The model under review builds one solid part; all positions refer to its coordinate system, in mm. A direction names the side the tool comes from. Give positions to 0.01 mm unless a question says otherwise; leave off trailing zeros. Order: outer loops, then holes, each group sorted by start corner. A loop starts at its lowest first (then second) coordinate and runs counter-clockwise, first axis right, second up. Notation, with made-up numbers: (-25, 11) - (10, 11) arc R28 cw to (10, 43) - close; hole circle Ø7 at (11, 67.5). An arc over 180 degrees is marked (long way). Use CSV: the item, a comma, the result in double quotes. Start each with the question number.
1. Machinability: for faces 1 (the flat face through (-0.635, 8, 0)), 2 (the flat face through (22.86, 18.7, -1.4)), 3 (the flat face through (-0.009, 8.219, -1.134)), 4 (the flat face through (44, 16.243, 3)), which of the approach directions +Z, -Z, +X, -X, +Y, -Y give a long, thin tool a straight path to every point of the face, cutting with its end or side? Answer none if there is none.
2. To check wall thickness, follow line 1 (X direction, y = 8.75, z = -0.25) (3 decimals); line 2 (X direction, y = 14, z = 2); line 3 (Z direction, x = 23, y = 8) (3 decimals). State the ranges of each line that lie inside material, in increasing order. Write a range as [from, to].
3. Take a section at A-A, the plane x = 41. State the section outline as (y, z) points (3 decimals), then the cut area to 3 significant figures.
4. Take a section at B-B, the plane y = 9.5. State the section outline as (x, z) points (3 decimals), then the cut area to 3 significant figures.
5. Take a section at C-C, the plane y = 13. State the section outline as (x, z) points (3 decimals).
6. For pin 1 (1.5 mm diameter, centred on x = 7, y = 19, fed in from +Z) (3 decimals); pin 2 (1.5 mm diameter, centred on x = 10.5, y = 16, fed in from -Z) (3 decimals); pin 3 (2 mm diameter, centred on y = 12, z = 3, fed in from -X); pin 4 (1.3 mm diameter, centred on y = 11.5, z = 2.5, fed in from +X), all flat-tipped, find the tip position at first contact; note any pin that passes through.
7. Take a section at D-D, the plane x = 15. State the section outline as (y, z) points (3 decimals).
8. Draft analysis for pull direction X (two halves, no side actions). For faces 5 (the flat face through (51, 5.715, -1.3)), 6 (the cylindrical face through (52.385, 8.084, 3.54)), 7 (the cylindrical face through (25.053, 20.635, 3.54)), state which applies: released by +X, released by -X, zero draft, split by the parting line, or undercut.
Autodesk Inventor part; units mm, degrees
ref_plane "YZ Plane" through (0, 0, 0) normal (1, 0, 0) x (0, 1, 0)
ref_plane "XZ Plane" through (0, 0, 0) normal (0, 1, 0) x (-1, 0, 0)
ref_plane "XY Plane" through (0, 0, 0) normal (0, 0, 1) x (1, 0, 0)
sketch "Sketch1" plane through (0, 0, 0) normal (0, 0, 1) x (1, 0, 0)
  line L0 (0, 0) -> (50.8, 0)
  line L1 (50.8, 0) -> (50.8, 19.05)
  line L2 (50.8, 19.05) -> (0, 19.05)
  line L3 (0, 19.05) -> (0, 0)
  line L4 (0, 0) -> (0, -2.54)
  line L5 (0, -2.54) -> (-2.54, -2.54)
  line L6 (-2.54, -2.54) -> (-2.54, 19.05)
  line L7 (-2.54, 19.05) -> (-2.54, 21.59)
  line L8 (-2.54, 21.59) -> (53.34, 21.59)
  line L9 (53.34, 21.59) -> (53.34, -2.54)
  line L10 (53.34, -2.54) -> (0, -2.54)
  dimension "d0" = 50.8
  dimension "d1" = 19.05
  dimension "d2" = 50.8
  dimension "d3" = 2.54
  dimension "d4" = 2.54
  dimension "d5" = 2.54
  dimension "d6" = 55.88
extrude "Extrusion1" add sketch "Sketch1" along normal blind 1.905
sketch "Sketch2" plane through (0, 0, 1.905) normal (0, 0, 1) x (1, 0, 0)
  line L0 (-2.54, -2.54) -> (-2.54, 21.59)
  line L1 (-2.54, 21.59) -> (53.34, 21.59)
  line L2 (53.34, 21.59) -> (-2.54, 21.59)
  line L3 (53.34, 21.59) -> (53.34, -2.54)
  line L4 (53.34, -2.54) -> (-2.54, -2.54)
  line L5 (-2.54, -2.54) -> (53.34, -2.54)
  point P0 (0, 0)
extrude "Extrusion2" add sketch "Sketch2" along normal blind 2.54
sketch "Sketch3" plane through (0, 0, 0) normal (0, 0, -1) x (-1, 0, 0)
  line L0 (0, 0) -> (2.54, 0)
  line L1 (2.54, 21.59) -> (2.54, -2.54)
  line L2 (2.54, 0) -> (2.54, 19.05)
  line L3 (2.54, 0) -> (0.635, 0)
  line L4 (0.635, 0) -> (0.635, 19.05)
  line L5 (0.635, 19.05) -> (0, 19.05)
  line L6 (0, 19.05) -> (0, 0)
  line L7 (0, 0) -> (-50.8, 0)
  line L8 (0, 19.05) -> (0.635, 19.05)
  line L9 (-50.8, 0) -> (-51.435, 0)
  line L10 (-51.435, 0) -> (-51.435, 19.05)
  line L11 (-51.435, 19.05) -> (-50.8, 19.05)
  line L12 (-50.8, 19.05) -> (-50.8, 0)
  dimension "d11" = 1.905
  dimension "d12" = 0.635
  dimension "d13" = 19.05
extrude "Extrusion3" cut sketch "Sketch3" against normal blind 1.905
sketch "Sketch4" plane through (0, 0, 0) normal (0, 0, -1) x (-1, 0, 0)
  line L0 (2.54, -2.54) -> (-53.34, -2.54)
  line L1 (0, 0) -> (-51.435, 0)
  line L2 (-51.435, 0) -> (-51.435, 19.05)
  line L3 (-51.435, 0) -> (-51.435, -2.54)
  line L4 (-51.435, -2.54) -> (0, -2.54)
  line L5 (0.635, 0) -> (0.635, -2.54)
  line L6 (0.635, 0) -> (0, 0)
  line L7 (0.635, 0) -> (-51.435, 0)
  line L8 (0.635, -2.54) -> (0, -2.54)
extrude "Extrusion4" cut sketch "Sketch4" against normal blind 1.905
sketch "Sketch5" plane through (0, 0, 4.445) normal (0, 0, 1) x (1, 0, 0)
  line L0 (-2.54, 21.59) -> (7.62, 21.59)
  line L1 (53.34, 21.59) -> (-2.54, 21.59)
  line L2 (7.62, 21.59) -> (7.62, 11.43)
  line L3 (-2.54, 21.59) -> (5.08, 21.59)
  line L4 (5.08, 21.59) -> (5.08, 13.97)
  line L5 (5.08, 13.97) -> (7.62, 13.97)
  line L6 (5.08, 13.97) -> (5.08, 11.43)
  line L7 (5.08, 11.43) -> (7.62, 11.43)
  line L8 (-2.54, 21.59) -> (26.67, 21.59)
  line L9 (-2.54, 21.59) -> (19.05, 21.59)
  line L10 (19.05, 10.795) -> (26.67, 10.795)
  line L11 (26.67, 18.415) -> (19.05, 18.415)
  line L12 (26.67, 21.59) -> (29.21, 21.59)
  line L13 (19.05, 21.59) -> (21.59, 21.59)
  line L14 (21.59, 10.795) -> (29.21, 10.795)
  line L15 (29.21, 10.795) -> (29.21, 21.59)
  line L16 (26.67, 18.415) -> (29.21, 18.415)
  line L17 (21.59, 21.59) -> (21.59, 18.415)
  line L18 (29.21, 18.415) -> (21.59, 18.415)
  line L19 (21.59, 18.415) -> (21.59, 10.795)
  line L20 (53.34, 21.59) -> (40.64, 21.59)
  line L21 (40.64, 21.59) -> (40.64, 8.89)
  line L22 (53.34, 21.59) -> (47.625, 21.59)
  line L23 (47.625, 21.59) -> (47.625, 15.875)
  line L24 (47.625, 15.875) -> (40.64, 15.875)
  line L25 (47.625, 15.875) -> (47.625, 8.89)
  line L26 (47.625, 8.89) -> (40.64, 8.89)
  point P0 (0, 0)
  dimension "d18" = 10.16
  dimension "d19" = 10.16
  dimension "d20" = 7.62
  dimension "d21" = 7.62
  dimension "d22" = 29.21
  dimension "d23" = 21.59
  dimension "d24" = 10.795
  dimension "d25" = 3.175
  dimension "d26" = 2.54
  dimension "d27" = 2.54
  dimension "d28" = 12.7
  dimension "d29" = 12.7
  dimension "d30" = 5.715
extrude "Extrusion5" cut sketch "Sketch5" against normal blind 2.54 contours L5 L2 L7 L6 | L25 L26 L21 L24 | L15 L14 L10 L19 L11 L16
move faces "Move1" translate (0, -2.54, 0) faces at (26.67, 18.415, 3.5983)
move faces "Move2" translate (0, 0, -0.635) faces at (34.0783, 20.7433, 0)
sketch "Sketch6" plane through (53.34, 21.59, -0.635) normal (0, 0, -1) x (-1, 0, 0)
  line L0 (1.905, -2.54) -> (1.905, -13.335)
  line L1 (1.905, -24.13) -> (1.905, -2.54)
  line L2 (1.905, -13.335) -> (1.905, -10.795)
  line L3 (1.905, -13.335) -> (1.905, -15.875)
  line L4 (1.905, -15.875) -> (3.175, -15.875)
  line L5 (3.175, -15.875) -> (3.175, -10.795)
  line L6 (3.175, -10.795) -> (1.905, -10.795)
  line L7 (1.905, -2.54) -> (27.94, -2.54)
  line L8 (1.905, -2.54) -> (53.975, -2.54)
  line L9 (27.94, -2.54) -> (30.48, -2.54)
  line L10 (27.94, -2.54) -> (25.4, -2.54)
  line L11 (25.4, -2.54) -> (25.4, -3.81)
  line L12 (25.4, -3.81) -> (30.48, -3.81)
  line L13 (30.48, -3.81) -> (30.48, -2.54)
  line L14 (53.975, -2.54) -> (53.975, -13.335)
  line L15 (53.975, -2.54) -> (53.975, -24.13)
  line L16 (53.975, -13.335) -> (53.975, -10.795)
  line L17 (53.975, -10.795) -> (52.705, -10.795)
  line L18 (52.705, -10.795) -> (52.705, -15.875)
  line L19 (52.705, -15.875) -> (53.975, -15.875)
  line L20 (53.975, -15.875) -> (53.975, -10.795)
  point P0 (53.34, -21.59)
  dimension "d39" = 10.795
  dimension "d40" = 2.54
  dimension "d41" = 2.54
  dimension "d42" = 5.08
  dimension "d43" = 26.035
  dimension "d44" = 2.54
  dimension "d45" = 2.54
  dimension "d46" = 1.27
  dimension "d47" = 5.08
  dimension "d48" = 10.795
  dimension "d49" = 2.54
  dimension "d51" = 1.27
  dimension "d52" = 5.08
extrude "Extrusion6" add sketch "Sketch6" against normal blind 0.889
move faces "Move3" translate (0, 0, -0.381) faces at (26.2467, 20.7433, -0.635)
move faces "Move4" translate (0, 0, -0.762) faces at (24.5533, 20.7433, -1.016)
sketch "Sketch10" plane through (50.165, 10.795, 0.254) normal (0, 1, 0) x (1, 0, 0)
  line L0 (1.27, 2.032) -> (1.27, 0)
  line L1 (1.27, 2.032) -> (1.27, 0.762)
  line L2 (0, 2.032) -> (0, 0)
  line L3 (1.27, 0.762) -> (0, 2.032)
  line L4 (1.27, 0) -> (0, 0)
  line L5 (0, 2.032) -> (0, 0)
  line L6 (0, 0) -> (1.27, 0)
  line L7 (1.27, 0) -> (1.27, 0.762)
  point P0 (-50.165, 0.254)
  dimension "d70" = 1.27
extrude "Extrusion10" cut sketch "Sketch10" against normal blind 25.4
sketch "Sketch11" plane through (22.86, 17.78, 0.254) normal (-1, 0, 0) x (0, 0, 1)
  line L0 (-2.032, 1.27) -> (-0.762, 1.27)
  line L1 (-2.032, 1.27) -> (0, 1.27)
  line L2 (-2.032, 0) -> (-2.032, 1.27)
  line L3 (-0.762, 1.27) -> (-2.032, 0)
  line L4 (-2.032, 0) -> (0, 0)
  line L5 (-2.032, 0) -> (0, 0)
  line L6 (0, 0) -> (0, 1.27)
  line L7 (0, 1.27) -> (-0.762, 1.27)
  point P0 (-0.254, -17.78)
  dimension "d73" = 1.27
extrude "Extrusion11" cut sketch "Sketch11" against normal blind 6.35 contours L1 L6 L4 L3
sketch "Sketch12" plane through (-0.635, 5.715, 0.254) normal (0, -1, 0) x (1, 0, 0)
  line L0 (1.27, -2.032) -> (0, -2.032)
  line L1 (0, -2.032) -> (0, -0.762)
  line L2 (0, -2.032) -> (0, 0)
  line L3 (0, -0.762) -> (1.27, -2.032)
  line L4 (1.27, -2.032) -> (1.27, 0)
  line L5 (0, 0) -> (1.27, 0)
  line L6 (1.27, 0) -> (0, 0)
  line L7 (0, 0) -> (0, -0.762)
  point P0 (0.635, -0.254)
  dimension "d76" = 1.27
extrude "Extrusion12" cut sketch "Sketch12" against normal blind 6.35 contours L3 L2 L5 L4
sketch "Sketch13" plane through (0, 0, 4.445) normal (0, 0, 1) x (1, 0, 0)
  line L0 (53.34, -2.54) -> (53.34, 21.59)
  line L1 (53.34, 21.59) -> (44.1325, 21.59)
  line L2 (53.34, 21.59) -> (-2.54, 21.59)
  line L3 (44.1325, 21.59) -> (44.1325, 16.2433)
  line L4 (48.006, 12.3825) -> (48.006, 8.4963)
  line L5 (48.006, 8.4963) -> (40.259, 8.4963)
  line L6 (40.259, 8.4963) -> (40.259, 16.2433)
  line L7 (40.259, 16.2433) -> (48.006, 16.2433)
  line L8 (48.006, 16.2433) -> (48.006, 12.3825)
  point P0 (0, 0)
  dimension "d79" = 9.2075
  dimension "d82" = 3.8862
  dimension "d83" = 7.747
  dimension "d84" = 7.747
  dimension "d85" = 7.747
extrude "Extrusion13" cut sketch "Sketch13" against normal blind 6.35
fillet "Fillet1" radius 3.175 2 edges at (-2.54, 9.525, 4.445) (53.34, 9.525, 4.445)
fillet "Fillet2" radius 3.175 5 edges at (-1.6101, 21.59, 3.5151) (-2.54, 21.59, -0.254) (52.4101, 21.59, 3.5151) (53.34, 21.59, -0.254) (25.4, 21.59, 4.445)
chamfer "Chamfer1" distance 0.635 angle 45 8 edges at (25.4, 15.875, 4.445) (29.21, 13.335, 4.445) (25.4, 10.795, 4.445) (21.59, 13.335, 4.445) (6.35, 13.97, 4.445) (7.62, 12.7, 4.445) (6.35, 11.43, 4.445) (5.08, 12.7, 4.445)
properties part number "PIUIODaughterBoardCover"
Determined:
1,face 1,"none"
1,face 2,"-Z, -Y"
1,face 3,"-Y"
1,face 4,"+Z, -Z"
2,line 1,"x = [-2.54, -0.635], [51.435, 53.34]"
2,line 2,"x = [-2.45, 21.59], [29.21, 40.26], [48.01, 53.25]"
2,line 3,"z = [1.905, 4.445]"
3,outline,"(-2.54, 1.905) - (8.496, 1.905) - (8.496, 4.445) - (-2.54, 4.445) - close; (16.243, 1.905) - (19.05, 1.905) - (19.05, -1.778) - (21.59, -1.778) - (21.59, 1.27) arc R3.175 ccw to (18.415, 4.445) - (16.243, 4.445) - close"
3,area,"48.8 mm²"
4,outline,"(-2.54, -1.778) - (0.635, -1.778) - (-0.635, -0.508) - (-0.635, 1.905) - (40.259, 1.905) - (40.259, 4.445) - (0.635, 4.445) arc R3.175 ccw to (-2.54, 1.27) - close; (48.006, 1.905) - (51.435, 1.905) - (51.435, -0.508) - (50.165, -1.778) - (53.34, -1.778) - (53.34, 1.27) arc R3.175 ccw to (50.165, 4.445) - (48.006, 4.445) - close"
4,area,"134 mm²"
5,outline,"(-2.54, -1.778) - (-0.635, -1.778) - (-0.635, 1.905) - (5.08, 1.905) - (5.08, 3.81) - (4.445, 4.445) - (0.635, 4.445) arc R3.175 ccw to (-2.54, 1.27) - close; (7.62, 1.905) - (21.59, 1.905) - (21.59, 3.81) - (20.955, 4.445) - (8.255, 4.445) - (7.62, 3.81) - close; (29.21, 1.905) - (40.259, 1.905) - (40.259, 4.445) - (29.845, 4.445) - (29.21, 3.81) - close; (48.006, 1.905) - (51.435, 1.905) - (51.435, -1.778) - (53.34, -1.778) - (53.34, 1.27) arc R3.175 ccw to (50.165, 4.445) - (48.006, 4.445) - close"
6,pin 1,"stops at z = 4.445"
6,pin 2,"stops at z = 1.905"
6,pin 3,"stops at x = -2.45"
6,pin 4,"stops at x = 53.29"
7,outline,"(-2.54, 1.905) - (19.05, 1.905) - (19.05, -1.778) - (21.59, -1.778) - (21.59, 1.27) arc R3.175 ccw to (18.415, 4.445) - (-2.54, 4.445) - close"
8,face 5,"undercut"
8,face 6,"released by +X"
8,face 7,"zero draft"
